```python
from build123d import *

# Parameters (mm, degrees)
SWEEP1_PROFILE_R = 0.5


with BuildPart() as part:
    # Sweep1: sweep along a path in Schizzo39
    with BuildLine(Plane.XY) as sweep1_path:
        Line((0, 0), (0, 5))
        Line((0, 5), (34.641016151, 25))
        Line((34.641016151, 25), (34.641016151, 35))
        Line((34.641016151, 35), (-10.358983849, 35))
        Line((-10.358983849, 35), (-10.358983849, 50))
        Line((-10.358983849, 50), (32.942286341, 75))
        Line((32.942286341, 75), (32.942286341, 90))
        Line((32.942286341, 90), (-27.057713659, 90))
        Line((-27.057713659, 90), (-22.057713659, 98.660254038))
        Line((-22.057713659, 98.660254038), (2.942286341, 98.660254038))
    # Sweep1 profile (on start of the path) → Sweep1 (sweep)
    with BuildSketch(Plane.ZX):
        Circle(SWEEP1_PROFILE_R)
    sweep(path=sweep1_path.line, transition=Transition.RIGHT)


solid = part.part
```
Here's how the part is built. I have some questions about the finished solid (model axes, mm). Round coordinates to 2 decimals unless told otherwise and drop trailing zeros. Order: outer loops, then holes, each group sorted by start corner. A loop starts at its lowest first (then second) coordinate and runs counter-clockwise, first axis right, second up. Notation, with made-up numbers: M 68.25,81 L 102.25,81 A26 ccw 102.25,107 Z; hole C 23,-1 d5. An arc over 180 degrees is marked long. Answer in a Markdown table with one row per item.
Item 1: Imagine slicing it at D-D, the plane x = 14. State how many separate pieces and enclosed holes the cut face has, and give its area (3 significant figures).
A:
| item | result |
|---|---|
| separate pieces | 4 |
| enclosed holes | 0 |
| area | 3.38 mm2 |
Item 2: Imagine slicing it at C-C, the plane y = 46. Write out the boundary of the cut face in (x, z), and give its area (3 significant figures).
A:
| item | result |
|---|---|
| outline | C -10.36,0 d1 |
| area | 0.785 mm2 |
Item 3: If I drill on L1, parallel to Y at x = 3.5, z = 0.05; L2, parallel to Y at x = -14.5, z = 0.1; L3, parallel to Y at x = 2.5, z = -0.4, over which ranges is the centre line in solid material (lowest first)? Write a range as from..to.
A:
| item | result |
|---|---|
| L1 | y = 6.45..7.6, 34.5..35.5, 57.43..58.58, 89.5..90.5 |
| L2 | y = 89.51..90.49, 98.17..99.15 |
| L3 | y = 6.1..6.79, 34.7..35.3, 57.08..57.77, 89.7..90.3, 98.36..98.96 |
Item 4: Imagine slicing it at B-B, the plane x = -20. Write out the boundary of the cut face in (y, z).
A:
| item | result |
|---|---|
| outline | C 90,0 d1; C 98.66,0 d1 |
Item 5: Imagine slicing it at A-A, the plane z = 0. Write out the boundary of the cut face in (x, y).
A:
| item | result |
|---|---|
| outline | M -27.92,89.5 L 32.44,89.5 L 32.44,75.29 L -10.86,50.29 L -10.86,34.5 L 34.14,34.5 L 34.14,25.29 L -0.5,5.29 L -0.5,0 L 0.5,0 L 0.5,4.71 L 35.14,24.71 L 35.14,35.5 L -9.86,35.5 L -9.86,49.71 L 33.44,74.71 L 33.44,90.5 L -26.19,90.5 L -21.77,98.16 L 2.94,98.16 L 2.94,99.16 L -22.35,99.16 Z |
